Source: CAD feature listing. Evaluate the final solid. Frame: model axes, mm. Face numbers are marked on the shaded views. A direction names the side the tool comes from. Give positions to 0.01 mm unless a question says otherwise; leave off trailing zeros. Order: outer loops, then holes, each group sorted by start corner. A loop starts at its lowest first (then second) coordinate and runs counter-clockwise, first axis right, second up.
1) Section D-D, the plane z = -2. Return loops of the section in (x, y).
2) Material intervals for line 1 (Z direction, x = 20.5, y = -9); line 2 (Y direction, x = 25, z = -8.25); line 3 (X direction, y = -11, z = -3.75), sorted ascending.
3) First-contact query: P1, Ø1.2, axis at x = 22, y = -15, coming from the -Z side; P2, Ø1.2, axis at x = 22.5, y = -9.5, coming from the -Z side; P3, Ø4, axis at x = 23, z = -11, coming from the -Y side; P4, Ø3.5, axis at x = 26.5, y = -18.5, coming from the -Z side. Flat tips, straight axial feed; report the tip coordinate or a pass-through.
4) Draft query along Z for the marked faces 5, 6 and 7. Return one class per face: released by +Z, released by -Z, zero draft, split by the parting line, or undercut.
5) Access query for the marked faces 1, 2, 3 and 4. Directions: +Z, -Z, +X, -X, +Y, -Y. A direction counts if a zero-diameter tool reaches every point of the face in a straight line with its end or side. Return the directions, or none.
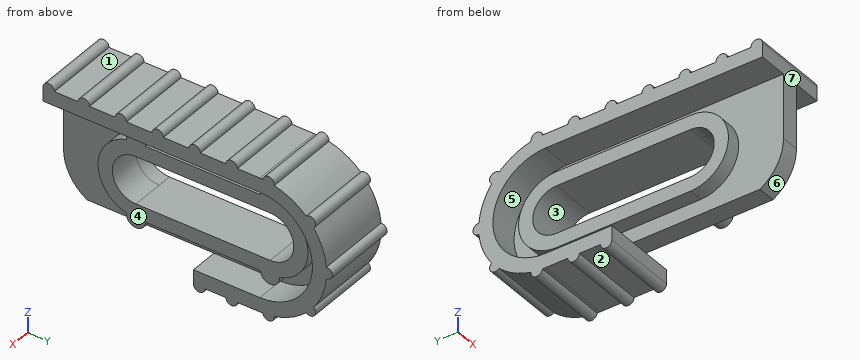
```python
from build123d import *

# Parameters (mm, degrees)
PAD104_DEPTH            = 1.9
POCKET097_DEPTH         = 2
PAD105_DEPTH            = 1.5
PAD106_DEPTH            = 1.5
PAD107_DEPTH            = 4.9
PAD108_DEPTH            = 3.1
PAD110_DEPTH            = 8
SKETCH201_R             = 1
PAD160_DEPTH            = 2
BODY016_ROLL_ANGLE      = -90
BODY016_PLACEMENT_ANGLE = 90


with BuildPart() as part:
    # Sketch196 → Pad104 (new body)
    with BuildSketch(Plane.XY):
        with BuildLine():
            Line((19.17, -5.55), (42.05, -5.55))
            ThreePointArc((42.05, -5.55), (47.6, 0), (42.05, 5.55))
            Line((21.65, 5.55), (42.05, 5.55))
            ThreePointArc((21.65, 5.55), (19.834103, 3.721462), (19.17, 1.231482))
            Line((19.17, -5.55), (19.17, 1.231482))
        make_face()
    extrude(amount=PAD104_DEPTH)

    # Sketch197 (on Face7 of Pad104) → Pocket097 (cut)
    with BuildSketch(Plane.XY.offset(1.9)):
        with BuildLine():
            ThreePointArc((27.9, 2.5), (25.4, 0), (27.9, -2.5))
            Line((27.9, -2.5), (42.05, -2.5))
            ThreePointArc((42.05, -2.5), (44.55, 0), (42.05, 2.5))
            Line((27.9, 2.5), (42.05, 2.5))
        make_face()
    extrude(amount=-POCKET097_DEPTH, mode=Mode.SUBTRACT)

    # Sketch198 (on Face5 of Pocket097) → Pad105 (join)
    with BuildSketch(Plane.XY.offset(1.9)):
        with BuildLine():
            ThreePointArc((42.05, -4), (46.05, 0), (42.05, 4))
            Line((27.9, 4), (42.05, 4))
            ThreePointArc((27.9, 4), (23.899997, 0), (27.9, -4))
            Line((42.05, -4), (27.9, -4))
        make_face()
        with BuildLine():
            ThreePointArc((27.9, 2.5), (25.399983, 0), (27.9, -2.5))
            Line((42.05, -2.5), (27.9, -2.5))
            ThreePointArc((42.05, -2.5), (44.55, 0), (42.05, 2.5))
            Line((42.05, 2.5), (27.9, 2.5))
        make_face(mode=Mode.SUBTRACT)
    extrude(amount=PAD105_DEPTH)

    # Sketch199 (on Face4 of Pad105) → Pad106 (join)
    with BuildSketch(Plane(origin=(0, 0, 0), x_dir=(1, 0, 0), z_dir=(0, 0, -1))):
        with BuildLine():
            Line((27.9, 4), (42.05, 4))
            ThreePointArc((42.05, -4), (46.050003, 0), (42.05, 4))
            Line((42.05, -4), (27.9, -4))
            ThreePointArc((27.9, 4), (23.899975, 0), (27.9, -4))
        make_face()
        with BuildLine():
            ThreePointArc((27.9, 2.5), (25.4, 0), (27.9, -2.5))
            Line((42.05, -2.5), (27.9, -2.5))
            ThreePointArc((42.05, -2.5), (44.55, 0), (42.05, 2.5))
            Line((27.9, 2.5), (42.05, 2.5))
        make_face(mode=Mode.SUBTRACT)
    extrude(amount=PAD106_DEPTH)

    # Sketch200 (on Face5 of Pad106) → Pad107 (join)
    with BuildSketch(Plane.XY.offset(1.9)):
        with BuildLine():
            ThreePointArc((42.05, -5.55), (47.6, 0), (42.05, 5.55))
            Line((42.05, 5.55), (35.05, 5.55))
            Line((35.05, 7.05), (35.05, 5.55))
            Line((42.05, 7.05), (35.05, 7.05))
            ThreePointArc((42.05, -7.05), (49.1, 0), (42.05, 7.05))
            Line((42.05, -7.05), (19.17, -7.05))
            Line((19.17, -7.05), (19.17, -5.55))
            Line((19.17, -5.55), (42.05, -5.55))
        make_face()
    extrude(amount=-PAD107_DEPTH)

    # Sketch200 (on Face5 of Pad106) → Pad108 (join)
    with BuildSketch(Plane.XY.offset(1.9)):
        with BuildLine():
            ThreePointArc((42.05, -5.55), (47.6, 0), (42.05, 5.55))
            Line((42.05, 5.55), (35.05, 5.55))
            Line((35.05, 7.05), (35.05, 5.55))
            Line((42.05, 7.05), (35.05, 7.05))
            ThreePointArc((42.05, -7.05), (49.1, 0), (42.05, 7.05))
            Line((42.05, -7.05), (19.17, -7.05))
            Line((19.17, -7.05), (19.17, -5.55))
            Line((19.17, -5.55), (42.05, -5.55))
        make_face()
    extrude(amount=PAD108_DEPTH)

    # Sketch202 → Pad110 (join)
    with BuildSketch(Plane(origin=(0, 0, -3), x_dir=(1, 0, 0), z_dir=(0, 0, -1))):
        with BuildLine():
            ThreePointArc((24.076013, 7.05), (23.476013, 7.65), (22.876013, 7.05))
            Line((22.876013, 7.05), (24.076013, 7.05))
        make_face()
        with BuildLine():
            ThreePointArc((27.976013, 7.05), (27.376013, 7.65), (26.776013, 7.05))
            Line((26.776013, 7.05), (27.976013, 7.05))
        make_face()
        with BuildLine():
            ThreePointArc((31.876013, 7.05), (31.276013, 7.65), (30.676013, 7.05))
            Line((30.676013, 7.05), (31.876013, 7.05))
        make_face()
        with BuildLine():
            ThreePointArc((35.776013, 7.05), (35.176013, 7.65), (34.576013, 7.05))
            Line((34.576013, 7.05), (35.776013, 7.05))
        make_face()
        with BuildLine():
            ThreePointArc((39.676013, 7.05), (39.076013, 7.65), (38.476013, 7.05))
            Line((38.476013, 7.05), (39.676013, 7.05))
        make_face()
        with BuildLine():
            ThreePointArc((49.074468, -0.599457), (49.7, 0), (49.074468, 0.599457))
            Line((49.074468, 0.599457), (49.074468, -0.599457))
        make_face()
        with BuildLine():
            ThreePointArc((47.727552, 4.179462), (47.802815, 5.042581), (46.937275, 5.081047))
            Line((46.937275, 5.081047), (47.727552, 4.179462))
        make_face()
        with BuildLine():
            ThreePointArc((43.564592, 6.885384), (43.052255, 7.584061), (42.376013, 7.042458))
            Line((42.376013, 7.042458), (43.564592, 6.885384))
        make_face()
        with BuildLine():
            ThreePointArc((46.937275, -5.081047), (47.802815, -5.042581), (47.727552, -4.179462))
            Line((47.727552, -4.179462), (46.937275, -5.081047))
        make_face()
        with BuildLine():
            ThreePointArc((42.376013, -7.042458), (43.052255, -7.584061), (43.564592, -6.885384))
            Line((43.564592, -6.885384), (42.376013, -7.042458))
        make_face()
        with BuildLine():
            ThreePointArc((38.476013, -7.05), (39.076013, -7.65), (39.676013, -7.05))
            Line((39.676013, -7.05), (38.476013, -7.05))
        make_face()
        with BuildLine():
            ThreePointArc((20.37, 7.05), (19.77, 7.65), (19.17, 7.05))
            Line((19.17, 7.05), (20.37, 7.05))
        make_face()
        with BuildLine():
            ThreePointArc((35.05, -7.05), (35.65, -7.65), (36.25, -7.05))
            Line((36.25, -7.05), (35.05, -7.05))
        make_face()
    extrude(amount=-PAD110_DEPTH)

    # Sketch201 (on Face19 of Pad108) → Pad160 (join)
    with BuildSketch(Plane(origin=(0, 0, -1.5), x_dir=(1, 0, 0), z_dir=(0, 0, -1))):
        with Locations((27.9, 4)):
            Circle(SKETCH201_R)
        with Locations((42.05, 4)):
            Circle(SKETCH201_R)
        with Locations((42.05, -4)):
            Circle(SKETCH201_R)
        with Locations((27.9, -4)):
            Circle(SKETCH201_R)
    extrude(amount=-PAD160_DEPTH)


with BuildPart() as part_1:
    # Body016 roll: moved
    add(part.part.rotate(Axis((0, 0, 0), (1, 0, 0)), BODY016_ROLL_ANGLE))


with BuildPart() as part_2:
    # Body016 placement: moved
    add(part_1.part.moved(Location((24.7, -51, -6.5))).rotate(Axis((24.7, -51, -6.5), (0, 0, 1)), BODY016_PLACEMENT_ANGLE))


solid = part_2.part
```
From the geometry:
1. outline: (19.7, -5.7) - (22.8, -5.7) - (22.8, -31.83) - (24.7, -31.83) - (24.7, -23.97) - (26.2, -23.97) - (26.2, -22.23) - (24.7, -22.23) - (24.7, -9.82) - (26.2, -9.82) - (26.2, -8.08) - (24.7, -8.08) - (24.7, -5.7) - (27.7, -5.7) - (27.7, -3.07) - (19.7, -3.07) - close
2. line 1: z = -13.55 to -12.05, -0.95 to 0.55
2. line 2: y = -26.7 to -24.89, -7.16 to -5.35, -3.68 to -2.12
2. line 3: x = 21.3 to 26.2
3. P1: stops at z = -14.15
3. P2: stops at z = -13.55
3. P3: stops at y = -31.67
3. P4: stops at z = -10.5
4. face 5: undercut
4. face 6: released by -Z
4. face 7: zero draft
5. face 1: +Z, +X, -X
5. face 2: -Z, +X, -X
5. face 3: +X, -X
5. face 4: +X, -Y
